```python
from build123d import *

# Parameters (mm, degrees)
BOSS_EXTRUDE1_DEPTH                                  = 12.7
SKETCH16_R                                           = 10.16
CUT_EXTRUDE3_DEPTH                                   = 1
CUT_EXTRUDE3_DEPTH_BACK                              = 13.7
SKETCH17_W                                           = 57.912
SKETCH17_H                                           = 57.912
CUT_EXTRUDE4_DEPTH                                   = 5.08
CBORE_FOR_3_8_BINDING_HEAD_MACHINE_SCREW_D           = 10.0838
CBORE_FOR_3_8_BINDING_HEAD_MACHINE_SCREW_CBORE_D     = 20.6375
CBORE_FOR_3_8_BINDING_HEAD_MACHINE_SCREW_CBORE_DEPTH = 10.7442
FILLET3_R                                            = 2.54
TAP_DRILL_FOR_10_24_TAP1_D                           = 3.7973
SKETCH24_R                                           = 19.1135
CUT_EXTRUDE5_DEPTH                                   = 1.778
FILLET4_R                                            = 2.54


with BuildPart() as part:
    # Sketch1 → Boss-Extrude1 (new body)
    with BuildSketch(Plane.XY):
        with BuildLine():
            Line((-35.173578353, -35.173578353), (35.173578353, -35.173578353))
            Line((35.173578353, -35.173578353), (35.173578353, -17.806510321))
            ThreePointArc((35.173578353, -17.806510321), (41.7, -6.708000046), (35.173578353, 4.390510229))
            Line((35.173578353, 4.390510229), (35.173578353, 35.173578353))
            Line((35.173578353, 35.173578353), (-35.173578353, 35.173578353))
            Line((-35.173578353, 35.173578353), (-35.173578353, 4.390510229))
            ThreePointArc((-35.173578353, 4.390510229), (-41.7, -6.708000046), (-35.173578353, -17.806510321))
            Line((-35.173578353, -17.806510321), (-35.173578353, -35.173578353))
        make_face()
    extrude(amount=BOSS_EXTRUDE1_DEPTH)

    # Sketch16 → Cut-Extrude3 (cut, two sides)
    with BuildSketch(Plane.XY.offset(12.7)) as cut_extrude3_sk:
        Circle(SKETCH16_R)
    extrude(amount=CUT_EXTRUDE3_DEPTH, mode=Mode.SUBTRACT)
    extrude(cut_extrude3_sk.sketch, amount=-CUT_EXTRUDE3_DEPTH_BACK, mode=Mode.SUBTRACT)

    # Sketch17 → Cut-Extrude4 (cut)
    with BuildSketch(Plane.XY.offset(12.7)):
        Rectangle(SKETCH17_W, SKETCH17_H)
    extrude(amount=-CUT_EXTRUDE4_DEPTH, mode=Mode.SUBTRACT)

    # CBORE for 3/8 Binding Head Machine Screw1 (through all)
    with Locations(Plane.XY.offset(12.7)):
        with Locations((-29, -6.708000046), (29, -6.708000046)):
            CounterBoreHole(CBORE_FOR_3_8_BINDING_HEAD_MACHINE_SCREW_D / 2, CBORE_FOR_3_8_BINDING_HEAD_MACHINE_SCREW_CBORE_D / 2, CBORE_FOR_3_8_BINDING_HEAD_MACHINE_SCREW_CBORE_DEPTH)

    # Fillet3
    fillet3_edges = [part.edges().sort_by_distance(p)[0] for p in [
        (35.173578353, -35.173578353, 6.35),
        (-35.173578353, -35.173578353, 6.35),
        (-35.173578353, 35.173578353, 6.35),
        (35.173578353, 35.173578353, 6.35),
        (28.956, 28.956, 10.16),
        (28.956, -28.956, 10.16),
        (-28.956, -28.956, 10.16),
        (-28.956, 28.956, 10.16),
    ]]
    fillet(fillet3_edges, radius=FILLET3_R)

    # Tap Drill for #10-24 Tap1 (through all)
    with Locations(Plane.XY.offset(7.62)):
        with Locations((-23.5, -23.5), (-23.5, 23.5), (23.5, 23.5), (23.5, -23.5)):
            Hole(TAP_DRILL_FOR_10_24_TAP1_D / 2)

    # Sketch24 → Cut-Extrude5 (cut)
    with BuildSketch(Plane.XY.offset(7.62)):
        Circle(SKETCH24_R)
    extrude(amount=-CUT_EXTRUDE5_DEPTH, mode=Mode.SUBTRACT)

    # Fillet4
    fillet4_edges = [part.edges().sort_by_distance(p)[0] for p in [
        (35.173578353, 4.390510229, 6.35),
        (35.173578353, -17.806510321, 6.35),
        (-35.173578353, -17.806510321, 6.35),
        (-35.173578353, 4.390510229, 6.35),
    ]]
    fillet(fillet4_edges, radius=FILLET4_R)


solid = part.part
```
CAD build for the part. Positions are in the model's coordinates, mm. A direction names the side the tool comes from. Round coordinates to 2 decimals unless told otherwise and drop trailing zeros. Loops run counter-clockwise (first coordinate to the right, second up) from the corner with the lowest first, then second, coordinate; pieces in that order, holes last. Notation, with made-up numbers: (-36.75, 45) - (-32.75, 45) arc R12 ccw to (-32.75, 65) - close; hole circle Ø1 at (-32, 22.25). An arc over 180 degrees is marked (long way). Return JSON: item names as keys, results as strings. Group by question number.
Q1. Flat gauge pins, fed straight in: pin 1 Ø5.5 at (y, z) = (-21, 10.5) entering from +X; pin 2 Ø4 at (y, z) = (19.5, 7) entering from +X; pin 3 Ø22.5 at (x, y) = (-30, -7) entering from +Z; pin 4 Ø5 at (x, y) = (-16.5, 2.5) entering from +Z. Where does each tip first touch, or does it go through?
Q2. Band-saw the part on D-D on y = 9. Give the cut face in (x, z), plus the area to 3 significant figures.
Q3. Two-plate mould, pull along X, no slides. Class faces 1 (the face through (-26.85, -1.98, 1.956)), 2 (the face through (-23.963, -6.486, 0.964)), 3 (the face through (-41.7, -6.5, 6.3)), 4 (the face through (34.41, -34.45, 6.44)): +X half, -X half, draft (parallel to the pull), parting line (faces both ways), or undercut.
Q4. Tool access for faces 5 (the face through (0, -35.174, 6)), 6 (the face through (35.174, -26, 6)), 7 (the face through (-35.174, -26, 6)), 8 (the face through (0, 20, 7.62)), 9 (the face through (35.174, 19, 6)): list every direction of +Z, -Z, +X, -X, +Y, -Y with a clear straight run to the whole face (end or side of a thin tool).
Q5. Band-saw the part on C-C on y = -23.5. Give the cut face in (x, z), plus the area to 3 significant figures.
Q6. Band-saw the part on B-B on x = 0. Give the cut face in (y, z).
Q7. Drill centre lines: line 1 along X through (y, z) = (7, 12); line 2 along X through (y, z) = (2, 7); line 3 along Y through (x, z) = (-24, 2.5). Where is each one in solid material? Low to high. Write a range as [from, to].
Q8. Band-saw the part on A-A on z = 9.75. Give the cut face in (x, y).
Solutions:
{
 "1": {"pin 1": "stops at x = 35.36", "pin 2": "stops at x = 35.17", "pin 3": "stops at z = 12.7", "pin 4": "stops at z = 7.62"},
 "2": {"outline": "(-35.17, 0) - (-4.71, 0) - (-4.71, 5.84) - (-16.86, 5.84) - (-16.86, 7.62) - (-28.96, 7.62) - (-28.96, 12.7) - (-35.17, 12.7) - close; (4.71, 0) - (35.17, 0) - (35.17, 12.7) - (28.96, 12.7) - (28.96, 7.62) - (16.86, 7.62) - (16.86, 5.84) - (4.71, 5.84) - close", "area": "484 mm^2"},
 "3": {"face 1": "undercut", "face 2": "undercut", "face 3": "-X half", "face 4": "+X half"},
 "4": {"face 5": "+Z, -Z, +X, -X, -Y", "face 6": "+Z, -Z, +X, -Y", "face 7": "+Z, -Z, -X, -Y", "face 8": "+Z", "face 9": "+Z, -Z, +X, +Y"},
 "5": {"outline": "(-35.17, 0) - (-25.4, 0) - (-25.4, 7.62) - (-28.96, 7.62) - (-28.96, 12.7) - (-35.17, 12.7) - close; (-21.6, 0) - (21.6, 0) - (21.6, 7.62) - (-21.6, 7.62) - close; (25.4, 0) - (35.17, 0) - (35.17, 12.7) - (28.96, 12.7) - (28.96, 7.62) - (25.4, 7.62) - close", "area": "541 mm^2"},
 "6": {"outline": "(-35.17, 0) - (-10.16, 0) - (-10.16, 5.84) - (-19.11, 5.84) - (-19.11, 7.62) - (-28.96, 7.62) - (-28.96, 12.7) - (-35.17, 12.7) - close; (10.16, 0) - (35.17, 0) - (35.17, 12.7) - (28.96, 12.7) - (28.96, 7.62) - (19.11, 7.62) - (19.11, 5.84) - (10.16, 5.84) - close"},
 "7": {"line 1": "x = [-35.17, -28.96], [28.96, 35.17]", "line 2": "x = [-38.24, -34.54], [-23.46, -19.01], [19.01, 23.46], [34.54, 38.24]", "line 3": "y = [-35.17, -25.33], [-21.67, -15.73], [2.32, 21.67], [25.33, 35.17]"},
 "8": {"outline": "(-36.26, -17.13) arc R2.54 cw to (-35.17, -19.21) - (-35.17, -32.63) arc R2.54 ccw to (-32.63, -35.17) - (32.63, -35.17) arc R2.54 ccw to (35.17, -32.63) - (35.17, -19.21) arc R2.54 cw to (36.26, -17.13) arc R12.7 ccw to (36.26, 3.71) arc R2.54 cw to (35.17, 5.8) - (35.17, 32.63) arc R2.54 ccw to (32.63, 35.17) - (-32.63, 35.17) arc R2.54 ccw to (-35.17, 32.63) - (-35.17, 5.8) arc R2.54 cw to (-36.26, 3.71) arc R12.7 ccw to start; hole (-28.96, -26.42) arc R2.54 ccw to (-26.42, -28.96) - (26.42, -28.96) arc R2.54 ccw to (28.96, -26.42) - (28.96, -17.03) arc R10.32 ccw (long way) to (28.96, 3.61) - (28.96, 26.42) arc R2.54 ccw to (26.42, 28.96) - (-26.42, 28.96) arc R2.54 ccw to (-28.96, 26.42) - (-28.96, 3.61) arc R10.32 ccw (long way) to (-28.96, -17.03) - close"}
}
